The listing builds one solid part. Answer for the finished solid, in the listing's coordinates (mm). Face numbers are marked on the shaded views. A direction names the side the tool comes from. Coordinates: 2 decimals unless noted, no trailing zeros. Write each loop counter-clockwise with the first axis right and the second up, starting at its lowest first coordinate (ties: lowest second). Pieces come first, ordered by that corner, then holes.
(1) Which of the six approach directions +Z, -Z, +X, -X, +Y, -Y give full straight-line access (tool end or side, diameter ignored) to the marked faces 4 and 5?
(2) Given P1, Ø2, axis at x = 184, z = -3.5, coming from the -Y side; P2, Ø1, axis at x = 154, z = -18, coming from the -Y side; P3, Ø8, axis at x = 113.5, y = -13, coming from the +Z side, each flat-ended and moving along its own axis, determine where each tip first touches the part or whether it passes through.
(3) The part is cut by section B-B on x = 186.5. Determine the outline of the cut face in (y, z), plus the area to 3 significant figures.
(4) The part is cut by section A-A on x = 50. Determine the outline of the cut face in (y, z).
(5) Straight lines are drawn through the part: line 1 (Z direction, x = 83, y = 7); line 2 (Y direction, x = 79.5, z = -2.5); line 3 (Z direction, x = 27.5, y = -7). For each, find the intervals that lie inside material, in ascending order.
(6) For a pull along X with two mould halves and no side action, classify the marked faces 1, 2 and 3 as +X half, -X half, draft (parallel to the pull), parting line (faces both ways), or undercut.
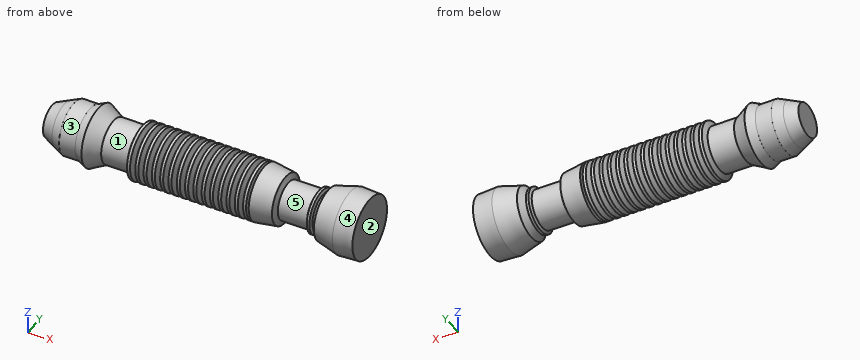
from build123d import *


# Not quite as in the source:
# - ends of sketch curves that miss each other by under 0.0002 mm in the source are joined


with BuildPart() as f1:
    # F0 (on Top) → F1 (revolve)
    with BuildSketch(Plane.XY):
        Polygon((146.7320563859, 15.8944390714), (152.7014625293, 15.8944390714), (150.8130326557, 20.0461714163), (149.7167594576, 20.0461714163), (148.6204862595, 20.0461714163), align=None)
        Polygon((0, 11.9488890163), (0, 0), (228.6, 0), (228.6, 22.225), (214.5352959633, 22.8744763881), (198.8992244005, 18.7337379903), (195.0535178185, 13.6998556554), (194.0553039312, 15.8944390714), (192.1773850918, 15.8944390714), (191.1042779684, 13.6998556554), (170.0893342495, 13.6998556554), (168.2125550841, 17.8259737997), (152.7014625293, 20.0461714163), (152.7014625293, 15.8944390714), (146.7320563859, 15.8944390714), (144.8436262557, 20.0461714163), (142.6510798595, 20.0461714163), (140.7626499859, 15.8944390714), (138.8742198557, 20.0461714163), (136.6816734595, 20.0461714163), (134.7932435859, 15.8944390714), (132.9048134557, 20.0461714163), (130.7122670595, 20.0461714163), (128.8238371859, 15.8944390714), (126.9354070557, 20.0461714163), (124.7428606595, 20.0461714163), (122.8544307859, 15.8944390714), (120.9660006557, 20.0461714163), (118.7734542595, 20.0461714163), (116.8850243859, 15.8944390714), (114.9965942557, 20.0461714163), (112.8040478595, 20.0461714163), (110.9156179859, 15.8944390714), (109.0271878557, 20.0461714163), (106.8346414595, 20.0461714163), (104.9462115859, 15.8944390714), (103.0577814557, 20.0461714163), (100.8652350595, 20.0461714163), (98.9768051859, 15.8944390714), (97.0883750557, 20.0461714163), (94.8958286595, 20.0461714163), (93.0073987859, 15.8944390714), (91.1189686557, 20.0461714163), (88.9264222595, 20.0461714163), (87.0379923859, 15.8944390714), (85.1495622557, 20.0461714163), (82.9570158595, 20.0461714163), (81.0685859859, 15.8944390714), (79.1801558557, 20.0461714163), (76.9876094595, 20.0461714163), (75.0991795859, 15.8944390714), (73.2107494557, 20.0461714163), (71.0182030595, 20.0461714163), (69.1297731859, 15.8944390714), (67.2413430557, 20.0461714163), (65.0487966595, 20.0461714163), (63.1603667859, 15.8944390714), (44.1223569214, 15.8944390714), (33.2462452351, 21.8172539027), (27.0914943445, 19.0177440883), (15.54095, 19.0177440883), (8.674332053, 15.8944390714), align=None)
    revolve(axis=Axis((114.3, 0, 0), (1, 0, 0)))


solid = f1.part
Model answer:
1. face 4: +X
1. face 5: none
2. P1: stops at y = -13.47
2. P2: stops at y = -9.4
2. P3: stops at z = 17.91
3. outline: circle Ø27.4 at (0, 0)
3. area: 590 mm2
4. outline: circle Ø31.79 at (0, 0)
5. line 1: z = -18.78 to 18.78
5. line 2: y = -19.18 to 19.18
5. line 3: z = -17.88 to 17.88
6. face 1: undercut
6. face 2: +X half
6. face 3: draft
